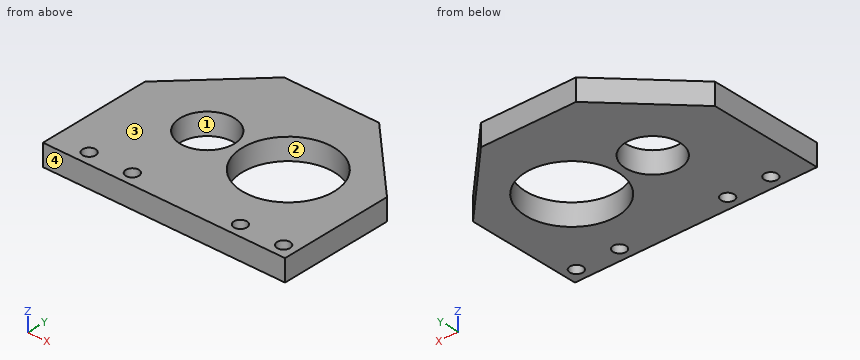
```python
from build123d import *

# Parameters (mm, degrees)
SKETCH1_W             = 71.12
SKETCH1_H             = 55.16372
SKETCH1_R             = 13.49375
SKETCH1_R_2           = 7.9375
BOSS_EXTRUDE1_DEPTH   = 6.35
F_6_CLEARANCE_HOLE1_D = 3.7973
CUT_EXTRUDE1_DEPTH    = 46.448818478


with BuildPart() as part:
    # Sketch1 → Boss-Extrude1 (new body)
    with BuildSketch(Plane.XY):
        Rectangle(SKETCH1_W, SKETCH1_H)
        with Locations((11.90625, 0)):
            Circle(SKETCH1_R, mode=Mode.SUBTRACT)
        with Locations((-11.90625, 0)):
            Circle(SKETCH1_R_2, mode=Mode.SUBTRACT)
    extrude(amount=BOSS_EXTRUDE1_DEPTH)

    # #6 Clearance Hole1 (through all)
    with Locations(Plane.XY.offset(6.35)):
        with Locations((-25.4, -23.77186), (-12.7, -23.77186), (19.05, -23.77186), (31.75, -23.77186)):
            Hole(F_6_CLEARANCE_HOLE1_D / 2)

    # Sketch4 → Cut-Extrude1 (cut, through all)
    with BuildSketch(Plane.XY.offset(6.35)):
        Polygon((-35.56, 5.99186), (-13.97, 27.58186), (-35.56, 27.58186), align=None)
        Polygon((35.56, 5.99186), (13.97, 27.58186), (35.56, 27.58186), align=None)
    extrude(amount=-CUT_EXTRUDE1_DEPTH, mode=Mode.SUBTRACT)


solid = part.part
```
Read the model definition and answer for the solid it produces. Units are mm, in the model's axes. Face numbers are marked on the shaded views. Give positions to 0.01 mm unless a question says otherwise; leave off trailing zeros. Order: outer loops, then holes, each group sorted by start corner. A loop starts at its lowest first (then second) coordinate and runs counter-clockwise, first axis right, second up. Notation, with made-up numbers: (83, 8) -> (121, 8) arc R22 cw to (121, 33) -> close; hole circle Ø7 at (15.25, 14). An arc over 180 degrees is marked (long way). Write item = value, one per line.
1. A cutting plane is placed at B-B, the plane x = -5. Write down the section's boundary in (y, z).
Numbers:
outline = (-27.58, 0) -> (-3.91, 0) -> (-3.91, 6.35) -> (-27.58, 6.35) -> close; (3.91, 0) -> (27.58, 0) -> (27.58, 6.35) -> (3.91, 6.35) -> close
2. A cutting plane is placed at D-D, the plane x = 19.05. Write down the section's boundary in (y, z).
Numbers:
outline = (-27.58, 0) -> (-25.67, 0) -> (-25.67, 6.35) -> (-27.58, 6.35) -> close; (-21.87, 0) -> (-11.45, 0) -> (-11.45, 6.35) -> (-21.87, 6.35) -> close; (11.45, 0) -> (22.5, 0) -> (22.5, 6.35) -> (11.45, 6.35) -> close
3. Given pin 1 (4.5 mm diameter, centred on x = 19.05, y = -23.77, fed in from -Z); pin 2 (3 mm diameter, centred on x = -27, z = 2.5, fed in from +Y); pin 3 (3.5 mm diameter, centred on x = -25.4, y = -23.77, fed in from -Z), each flat-ended and moving along its own axis, determine where each tip first touches the part or whether it passes through.
Numbers:
pin_1 = 0
pin_2 = 16.05
pin_3 = through
4. A cutting plane is placed at A-A, the plane y = 0. Write down the section's boundary in (x, z), and give its area (3 significant figures).
Numbers:
outline = (-35.56, 0) -> (-19.84, 0) -> (-19.84, 6.35) -> (-35.56, 6.35) -> close; (-3.97, 0) -> (-1.59, 0) -> (-1.59, 6.35) -> (-3.97, 6.35) -> close; (25.4, 0) -> (35.56, 0) -> (35.56, 6.35) -> (25.4, 6.35) -> close
area = 179 mm²
5. A cutting plane is placed at C-C, the plane y = -10. Write down the section's boundary in (x, z), and give its area (3 significant figures).
Numbers:
outline = (-35.56, 0) -> (2.85, 0) -> (2.85, 6.35) -> (-35.56, 6.35) -> close; (20.97, 0) -> (35.56, 0) -> (35.56, 6.35) -> (20.97, 6.35) -> close
area = 337 mm²
6. Straight lines are drawn through the part: line 1 along Y through (x, z) = (-12.7, 4); line 2 along Y through (x, z) = (19.05, 2.5); line 3 along X through (y, z) = (5.5, 3.75). For each, find the intervals that lie inside material, in ascending order.
Numbers:
line_1 = -27.58 to -25.67, -21.87 to -7.9, 7.9 to 27.58
line_2 = -27.58 to -25.67, -21.87 to -11.45, 11.45 to 22.5
line_3 = -35.56 to -17.63, -6.18 to -0.42, 24.23 to 35.56
7. The mould has two halves that part along Y. Classify the marked faces 1, 2, 3 and 4: +Y half, -Y half, draft (parallel to the pull), parting line (faces both ways), or undercut.
Numbers:
face_1 = undercut
face_2 = undercut
face_3 = draft
face_4 = -Y half
